Source: CAD feature listing. Evaluate the final solid. Frame: model axes, mm. Face numbers are marked on the shaded views. A direction names the side the tool comes from. Round coordinates to 2 decimals unless told otherwise and drop trailing zeros. Loops run counter-clockwise (first coordinate to the right, second up) from the corner with the lowest first, then second, coordinate; pieces in that order, holes last.
(1) Section B-B, the plane z = 8.5. Return the cut outline in (x, y), plus the area to 3 significant figures.
(2) Section D-D, the plane y = -3.25. Return the cut outline in (x, z).
(3) First-contact query: pin 1 Ø5 at (y, z) = (3, 25.5) entering from +X; pin 2 Ø6 at (x, y) = (17.78, 0) entering from -Z; pin 3 Ø4 at (x, y) = (-17, 1.5) entering from +Z; pin 4 Ø3 at (y, z) = (2.5, 19.5) entering from -X. Flat tips, straight axial feed; report the tip coordinate or a pass-through.
(4) Section A-A, the plane x = -17.78. Return the cut outline in (y, z), plus the area to 3 significant figures.
(5) Mould query, pull axis Y, two halves, no side actions, for the marked faces 1, 2, 3 and 4. Classes: pulls with the +Y half, pulls with the -Y half, needs draft (parallel to the pull), parting line crosses it, or undercut.
(6) Section C-C, the plane x = 5.08. Return the cut outline in (y, z).
(7) Material intervals for probe 1 along X at (y, z) = (0, 7.5); probe 2 along Y at (x, z) = (17.78, 9.5); probe 3 along X at (y, z) = (0.5, 15), sorted ascending.
(8) Set-up query: the marked faces 5, 6 and 7. Return all of +Z, -Z, +X, -X, +Y, -Y with unobstructed straight access to the full face (end or side cutting, diameter ignored); none if empty.
```python
from build123d import *

# Parameters (mm, degrees)
SKETCH1_W            = 48.26
SKETCH1_H            = 12.7
SKETCH1_R            = 2.54
BOSS_EXTRUDE2_DEPTH  = 5.08
SKETCH3_R            = 2.54
CUT_EXTRUDE1_DEPTH   = 6.08
SKETCH4_W            = 3.81
SKETCH4_H            = 12.7
BOSS_EXTRUDE5_DEPTH  = 27.94
SKETCH5_W            = 3.81
SKETCH5_H            = 12.7
BOSS_EXTRUDE6_DEPTH  = 27.94
SKETCH7_W            = 22.86
SKETCH7_H            = 12.7
BOSS_EXTRUDE8_DEPTH  = 2.032
SKETCH10_R           = 2.54
CUT_EXTRUDE4_DEPTH   = 2.032
SKETCH11_R           = 2.54
CUT_EXTRUDE5_DEPTH   = 2.032
FILLET12_R           = 2.54
SKETCH12_W           = 15.24
SKETCH12_H           = 12.7
BOSS_EXTRUDE9_DEPTH  = 27.94
SKETCH13_R           = 2.54
CUT_EXTRUDE6_DEPTH   = 7.493
SKETCH14_R           = 2.54
CUT_EXTRUDE7_DEPTH   = 7.493
SKETCH20_R           = 4.8006
CUT_EXTRUDE13_DEPTH  = 3.429
SKETCH21_W           = 12.7
SKETCH21_H           = 12.7
BOSS_EXTRUDE10_DEPTH = 20.32
SKETCH22_R           = 2.54
CUT_EXTRUDE14_DEPTH  = 20.32
SKETCH23_W           = 12.7
SKETCH23_H           = 12.7
BOSS_EXTRUDE11_DEPTH = 20.32
SKETCH24_R           = 2.54
CUT_EXTRUDE15_DEPTH  = 25.4
SKETCH26_R           = 4.8006
CUT_EXTRUDE16_DEPTH  = 3.429
FILLET15_R           = 2.38
FILLET16_R           = 2.38
FILLET17_R           = 2.38


with BuildPart() as part:
    # Sketch1 → Boss-Extrude2 (new body)
    with BuildSketch(Plane.XY):
        Rectangle(SKETCH1_W, SKETCH1_H)
        with Locations((-17.78, 0)):
            Circle(SKETCH1_R, mode=Mode.SUBTRACT)
    extrude(amount=-BOSS_EXTRUDE2_DEPTH)

    # Sketch3 → Cut-Extrude1 (cut, through all)
    with BuildSketch(Plane.XY):
        with Locations((17.78, 0)):
            Circle(SKETCH3_R)
    extrude(amount=-CUT_EXTRUDE1_DEPTH, mode=Mode.SUBTRACT)

    # Sketch4 → Boss-Extrude5 (add)
    with BuildSketch(Plane.XY):
        with Locations((-9.525, 0)):
            Rectangle(SKETCH4_W, SKETCH4_H)
    extrude(amount=BOSS_EXTRUDE5_DEPTH)

    # Sketch5 → Boss-Extrude6 (add)
    with BuildSketch(Plane.XY):
        with Locations((9.525, 0)):
            Rectangle(SKETCH5_W, SKETCH5_H)
    extrude(amount=BOSS_EXTRUDE6_DEPTH)

    # Sketch7 → Boss-Extrude8 (add)
    with BuildSketch(Plane.XY.offset(27.94)):
        Rectangle(SKETCH7_W, SKETCH7_H)
    extrude(amount=BOSS_EXTRUDE8_DEPTH)

    # Sketch10 → Cut-Extrude4 (cut)
    with BuildSketch(Plane.XY.offset(29.972)):
        with Locations((-5.08, 0)):
            Circle(SKETCH10_R)
    extrude(amount=-CUT_EXTRUDE4_DEPTH, mode=Mode.SUBTRACT)

    # Sketch11 → Cut-Extrude5 (cut)
    with BuildSketch(Plane.XY.offset(29.972)):
        with Locations((5.08, 0)):
            Circle(SKETCH11_R)
    extrude(amount=-CUT_EXTRUDE5_DEPTH, mode=Mode.SUBTRACT)

    # Fillet12
    fillet12_edges = [part.edges().sort_by_distance(p)[0] for p in [
        (-11.43, 0, 29.972),
        (11.43, 0, 29.972),
    ]]
    fillet(fillet12_edges, radius=FILLET12_R)

    # Sketch12 → Boss-Extrude9 (add)
    with BuildSketch(Plane.XY):
        Rectangle(SKETCH12_W, SKETCH12_H)
    extrude(amount=BOSS_EXTRUDE9_DEPTH)

    # Sketch13 → Cut-Extrude6 (cut)
    with BuildSketch(Plane.XY.offset(27.94)):
        with Locations((-5.08, 0)):
            Circle(SKETCH13_R)
    extrude(amount=-CUT_EXTRUDE6_DEPTH, mode=Mode.SUBTRACT)

    # Sketch14 → Cut-Extrude7 (cut)
    with BuildSketch(Plane.XY.offset(27.94)):
        with Locations((5.08, 0)):
            Circle(SKETCH14_R)
    extrude(amount=-CUT_EXTRUDE7_DEPTH, mode=Mode.SUBTRACT)

    # Sketch20 → Cut-Extrude13 (cut)
    with BuildSketch(Plane(origin=(0, 0, -5.08), x_dir=(-1, 0, 0), z_dir=(0, 0, -1))):
        with Locations((17.78, 0)):
            Circle(SKETCH20_R)
    extrude(amount=-CUT_EXTRUDE13_DEPTH, mode=Mode.SUBTRACT)

    # Sketch21 → Boss-Extrude10 (add)
    with BuildSketch(Plane.XY):
        with Locations((-17.78, 0)):
            Rectangle(SKETCH21_W, SKETCH21_H)
    extrude(amount=BOSS_EXTRUDE10_DEPTH)

    # Sketch22 → Cut-Extrude14 (cut)
    with BuildSketch(Plane(origin=(0, 0, 0), x_dir=(-1, 0, 0), z_dir=(0, 0, -1))):
        with Locations((17.78, 0)):
            Circle(SKETCH22_R)
    extrude(amount=-CUT_EXTRUDE14_DEPTH, mode=Mode.SUBTRACT)

    # Sketch23 → Boss-Extrude11 (add)
    with BuildSketch(Plane.XY):
        with Locations((17.78, 0)):
            Rectangle(SKETCH23_W, SKETCH23_H)
    extrude(amount=BOSS_EXTRUDE11_DEPTH)

    # Sketch24 → Cut-Extrude15 (cut)
    with BuildSketch(Plane(origin=(0, 0, -5.08), x_dir=(-1, 0, 0), z_dir=(0, 0, -1))):
        with Locations((-17.78, 0)):
            Circle(SKETCH24_R)
    extrude(amount=-CUT_EXTRUDE15_DEPTH, mode=Mode.SUBTRACT)

    # Sketch26 → Cut-Extrude16 (cut)
    with BuildSketch(Plane(origin=(0, 0, -5.08), x_dir=(-1, 0, 0), z_dir=(0, 0, -1))):
        with Locations((-17.78, 0)):
            Circle(SKETCH26_R)
    extrude(amount=-CUT_EXTRUDE16_DEPTH, mode=Mode.SUBTRACT)

    # Fillet15
    fillet15_edges = [part.edges().sort_by_distance(p)[0] for p in [
        (11.43, 0, 20.32),
    ]]
    fillet(fillet15_edges, radius=FILLET15_R)

    # Fillet16
    fillet16_edges = [part.edges().sort_by_distance(p)[0] for p in [
        (-11.43, 0, 20.32),
    ]]
    fillet(fillet16_edges, radius=FILLET16_R)

    # Fillet17
    fillet17_edges = [part.edges().sort_by_distance(p)[0] for p in [
        (-24.13, 0, 20.32),
        (24.13, 0, 20.32),
    ]]
    fillet(fillet17_edges, radius=FILLET17_R)


solid = part.part
```
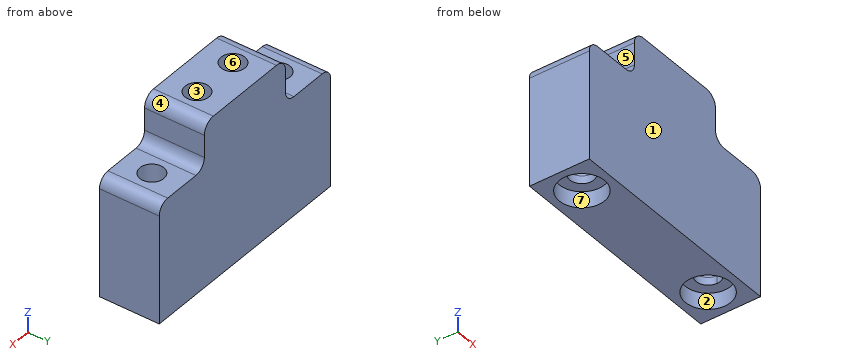
Output values:
1. outline: (-24.13, -6.35) - (24.13, -6.35) - (24.13, 6.35) - (-24.13, 6.35) - close; hole circle Ø5.08 at (-17.78, 0); hole circle Ø5.08 at (17.78, 0)
1. area: 572 mm2
2. outline: (-24.13, -5.08) - (-21.31, -5.08) - (-21.31, -1.65) - (-14.25, -1.65) - (-14.25, -5.08) - (14.25, -5.08) - (14.25, -1.65) - (21.31, -1.65) - (21.31, -5.08) - (24.13, -5.08) - (24.13, 17.94) arc R2.38 ccw to (21.75, 20.32) - (13.81, 20.32) arc R2.38 cw to (11.43, 22.7) - (11.43, 27.43) arc R2.54 ccw to (8.89, 29.97) - (-8.89, 29.97) arc R2.54 ccw to (-11.43, 27.43) - (-11.43, 22.7) arc R2.38 cw to (-13.81, 20.32) - (-21.75, 20.32) arc R2.38 ccw to (-24.13, 17.94) - close
3. pin 1: stops at x = 11.43
3. pin 2: stops at z = -1.65
3. pin 3: stops at z = 20.32
3. pin 4: stops at x = -24.13
4. outline: (-6.35, -5.08) - (-4.8, -5.08) - (-4.8, -1.65) - (-2.54, -1.65) - (-2.54, 20.32) - (-6.35, 20.32) - close; (2.54, -1.65) - (4.8, -1.65) - (4.8, -5.08) - (6.35, -5.08) - (6.35, 20.32) - (2.54, 20.32) - close
4. area: 178 mm2
5. face 1: pulls with the -Y half
5. face 2: undercut
5. face 3: undercut
5. face 4: needs draft
6. outline: (-6.35, -5.08) - (6.35, -5.08) - (6.35, 29.97) - (2.54, 29.97) - (2.54, 20.45) - (-2.54, 20.45) - (-2.54, 29.97) - (-6.35, 29.97) - close
7. probe 1: x = -24.13 to -20.32, -15.24 to 15.24, 20.32 to 24.13
7. probe 2: y = -6.35 to -2.54, 2.54 to 6.35
7. probe 3: x = -24.13 to -20.27, -15.29 to 15.29, 20.27 to 24.13
8. face 5: +Z, -X, +Y, -Y
8. face 6: +Z
8. face 7: -Z
